Here's how the part is built. I have some questions about the finished solid (model axes, mm). A direction names the side the tool comes from. Round coordinates to 2 decimals unless told otherwise and drop trailing zeros. Order: outer loops, then holes, each group sorted by start corner. A loop starts at its lowest first (then second) coordinate and runs counter-clockwise, first axis right, second up.
```python
from build123d import *

# Parameters (mm, degrees)
SKETCH_W        = 118
SKETCH_H        = 81
PAD_DEPTH       = 2
SKETCH001_R     = 1.7
HOLE_DEPTH      = 25
SKETCH002_W     = 12
SKETCH002_H     = 41
PAD001_DEPTH    = 15
SKETCH003_W     = 10
SKETCH003_H     = 39
POCKET_DEPTH    = 17.001
SKETCH004_W     = 27
SKETCH004_H     = 47
POCKET001_DEPTH = 5


with BuildPart() as part:
    # Sketch → Pad (new body)
    with BuildSketch(Plane.XY):
        Rectangle(SKETCH_W, SKETCH_H)
    extrude(amount=PAD_DEPTH)

    # Sketch001 (on Face5 of Pad) → Hole (cut)
    with BuildSketch(Plane(origin=(0, 0, 0), x_dir=(1, 0, 0), z_dir=(0, 0, -1))):
        with Locations((-48, 20.5)):
            Circle(SKETCH001_R)
        with Locations((-48, -20.5)):
            Circle(SKETCH001_R)
        with Locations((48, 20.5)):
            Circle(SKETCH001_R)
        with Locations((48, -20.5)):
            Circle(SKETCH001_R)
    extrude(amount=-HOLE_DEPTH, mode=Mode.SUBTRACT)

    # Sketch002 (on Face5 of Hole) → Pad001 (join)
    with BuildSketch(Plane.XY.offset(2)):
        with Locations((-2.5, 0)):
            Rectangle(SKETCH002_W, SKETCH002_H)
    extrude(amount=PAD001_DEPTH)

    # Sketch003 (on Face15 of Pad001) → Pocket (cut, through all)
    with BuildSketch(Plane.XY.offset(17)):
        with Locations((-2.5, 0)):
            Rectangle(SKETCH003_W, SKETCH003_H)
    extrude(amount=-POCKET_DEPTH, mode=Mode.SUBTRACT)

    # Sketch004 (on Face5 of Pocket) → Pocket001 (cut)
    with BuildSketch(Plane.XY.offset(2)):
        with Locations((-23.5, 0.180496)):
            Rectangle(SKETCH004_W, SKETCH004_H)
    extrude(amount=-POCKET001_DEPTH, mode=Mode.SUBTRACT)


solid = part.part
```
1. If we section it at A-A, the plane x = -24.5: Write out the boundary of the cut face in (y, z).
Evaluation:
outline: (-40.5, 0) - (-23.32, 0) - (-23.32, 2) - (-40.5, 2) - close; (23.68, 0) - (40.5, 0) - (40.5, 2) - (23.68, 2) - close
2. If we section it at B-B, the plane y = 12: Write out the boundary of the cut face in (x, z), and give its area (3 significant figures).
Evaluation:
outline: (-59, 0) - (-37, 0) - (-37, 2) - (-59, 2) - close; (-10, 0) - (-7.5, 0) - (-7.5, 17) - (-8.5, 17) - (-8.5, 2) - (-10, 2) - close; (2.5, 0) - (59, 0) - (59, 2) - (3.5, 2) - (3.5, 17) - (2.5, 17) - close
area: 192 mm2
3. If we section it at D-D, the plane x = -48: Write out the boundary of the cut face in (y, z), and give its area (3 significant figures).
Evaluation:
outline: (-40.5, 0) - (-22.2, 0) - (-22.2, 2) - (-40.5, 2) - close; (-18.8, 0) - (18.8, 0) - (18.8, 2) - (-18.8, 2) - close; (22.2, 0) - (40.5, 0) - (40.5, 2) - (22.2, 2) - close
area: 148 mm2
4. If we mould it in two halves opening along X, with no side actions, what happens to faces 1 (the flat face through (-7.5, 0, 9)), 2 (the flat face through (-3, 20.5, 9)), 3 (the flat face through (-8.5, 0, 9))? For each: released by +X, released by -X, zero draft, split by the parting line, or undercut.
Evaluation:
face 1: undercut
face 2: zero draft
face 3: released by -X
5. I'm going to push flat-ended pins straight in: P1, Ø5.5, axis at x = 48, y = -20.5, coming from the +Z side; P2, Ø4.5, axis at y = -10, z = 6, coming from the +X side; P3, Ø2.5, axis at x = -48, y = 20.5, coming from the +Z side (1 decimal); P4, Ø8, axis at x = -4, z = 12, coming from the +Y side. Where does each tip first touch, or does it pass through?
Evaluation:
P1: stops at z = 2
P2: stops at x = 3.5
P3: passes through
P4: stops at y = 20.5
6. I need wall thicknesses on probe 1 along Y at (x, z) = (-48, 1.55); probe 2 along X at (y, z) = (-20.5, 1.5); probe 3 along Y at (x, z) = (-6, 13.5). Which ranges of each line are inside material? Lowest first, please.
Evaluation:
probe 1: y = -40.5 to -22.2, -18.8 to 18.8, 22.2 to 40.5
probe 2: x = -59 to -49.7, -46.3 to -37, -10 to 46.3, 49.7 to 59
probe 3: y = -20.5 to -19.5, 19.5 to 20.5
7. If we section it at C-C, the plane z = 9.25: Write out the boundary of the cut face in (x, y).
Evaluation:
outline: (-8.5, -20.5) - (3.5, -20.5) - (3.5, 20.5) - (-8.5, 20.5) - close; hole (-7.5, -19.5) - (2.5, -19.5) - (2.5, 19.5) - (-7.5, 19.5) - close
8. On a 3-axis mill with a long thin cutter (end or side, diameter ignored), from which of +Z, -Z, +X, -X, +Y, -Y can I reach the whole of each face in a straight line? I mean faces 4 (the flat face through (-3, -19.5, 9)), 5 (the flat face through (-3, -20.5, 9)), 6 (the flat face through (3.5, 0, 9)). Say none if no direction works.
Evaluation:
face 4: +Z, -Z
face 5: +Z, +X, -X, -Y
face 6: +Z, +X, +Y, -Y
